```python
from build123d import *

# Parameters (mm, degrees)
F1_DEPTH = 7.5
F2_R     = 4
F3_T     = -0.95


with BuildPart() as f1:
    # F0 (on Top) → F1 (new body)
    with BuildSketch(Plane.XY):
        Polygon((-11.2561800848, -12.5999993347), (14, -12.5999993347), (14, 2.4000006653), (14, 8.4000006653), (14, 12.4000006653), (-14, 12.4000006653), (-14, 5.4000006653), (-14, -12.5999993347), align=None)
        with BuildLine():
            ThreePointArc((2.6457513111, -8.5999993347), (0, -9.5999993347), (-2.6457513111, -8.5999993347))
            Line((-2.6457513111, -8.5999993347), (-5.3542486889, -8.5999993347))
            ThreePointArc((-5.3542486889, -8.5999993347), (-8, -9.5999993347), (-10.6457513111, -8.5999993347))
            ThreePointArc((-10.6457513111, -8.5999993347), (-12, -5.5999993347), (-10.6457513111, -2.5999993347))
            ThreePointArc((-10.6457513111, -2.5999993347), (-8, -1.5999993347), (-5.3542486889, -2.5999993347))
            Line((-5.3542486889, -2.5999993347), (-2.6457513111, -2.5999993347))
            ThreePointArc((-2.6457513111, -2.5999993347), (0, -1.5999993347), (2.6457513111, -2.5999993347))
            Line((2.6457513111, -2.5999993347), (5.3542486889, -2.5999993347))
            ThreePointArc((5.3542486889, -2.5999993347), (8, -1.5999993347), (10.6457513111, -2.5999993347))
            ThreePointArc((10.6457513111, -2.5999993347), (12, -5.5999993347), (10.6457513111, -8.5999993347))
            ThreePointArc((10.6457513111, -8.5999993347), (8, -9.5999993347), (5.3542486889, -8.5999993347))
            Line((5.3542486889, -8.5999993347), (2.6457513111, -8.5999993347))
        make_face(mode=Mode.SUBTRACT)
        with BuildLine():
            Line((-2.6457513111, 2.4000006653), (-5.3542486889, 2.4000006653))
            ThreePointArc((-5.3542486889, 2.4000006653), (-12, 5.4000006653), (-5.3542486889, 8.4000006653))
            Line((-5.3542486889, 8.4000006653), (-2.6457513111, 8.4000006653))
            ThreePointArc((-2.6457513111, 8.4000006653), (0, 9.4000006653), (2.6457513111, 8.4000006653))
            Line((2.6457513111, 8.4000006653), (5.3542486889, 8.4000006653))
            ThreePointArc((5.3542486889, 8.4000006653), (8, 9.4000006653), (10.6457513111, 8.4000006653))
            ThreePointArc((10.6457513111, 8.4000006653), (12, 5.4000006653), (10.6457513111, 2.4000006653))
            ThreePointArc((10.6457513111, 2.4000006653), (8, 1.4000006653), (5.3542486889, 2.4000006653))
            Line((5.3542486889, 2.4000006653), (2.6457513111, 2.4000006653))
            ThreePointArc((2.6457513111, 2.4000006653), (0, 1.4000006653), (-2.6457513111, 2.4000006653))
        make_face(mode=Mode.SUBTRACT)
    extrude(amount=F1_DEPTH)

    # F2
    f2_edges = [f1.edges().sort_by_distance(p)[0] for p in [
        (-14, 12.400001, 3.75),
        (14, -12.599999, 3.75),
        (-14, -12.599999, 3.75),
        (14, 12.400001, 3.75),
    ]]
    fillet(f2_edges, radius=F2_R)

    # F3
    f3_openings = [f1.faces().sort_by_distance(p)[0] for p in [
        (0, -0.099999, 7.5),
    ]]
    offset(amount=F3_T, openings=f3_openings)


solid = f1.part
```
Work out the finished part from the listing and answer in its coordinate system (mm). A direction names the side the tool comes from. Coordinates: 2 decimals unless noted, no trailing zeros. Write each loop counter-clockwise with the first axis right and the second up, starting at its lowest first coordinate (ties: lowest second). Pieces come first, ordered by that corner, then holes.
Q1. A cutting plane is placed at B-B, the plane x = -8. Give the vertices of the cut face in (y, z).
Q2. A cutting plane is placed at A-A, the plane y = 5.4. Give the vertices of the cut face in (x, z), then the cut area to 3 significant figures.
Q3. Find the intervals of material crossed by line 1 (Y direction, x = 7.75, z = 5); line 2 (Y direction, x = -4.5, z = 5.75); line 3 (X direction, y = -0.25, z = 3.5), in increasing order.
Q4. A cutting plane is placed at C-C, the plane z = 0.5. Give the vertices of the cut face in (x, y), then the cut area to 3 significant figures.
Q5. Determine the mould class of faces 4 (the face through (-12.133, -10.78, 4.271)), 5 (the face through (0, -10, 7.5)), 6 (the face through (-12.797, 11.259, 3.802)), 7 (the face through (4, 8.4, 4)) for opening direction Y: released by +Y, released by -Y, zero draft, split by the parting line, or undercut.
Q6. This flat-tipped pin is pushed along its axis until it touches: pin 1 Ø1.5 at (y, z) = (9.5, 2.5) entering from -X. Where does it stop, or does it pass through?
Q7. A cutting plane is placed at D-D, the plane z = 3.75. State how many separate pieces and enclosed holes the cut face has, then the cut area to 3 significant figures.
Q8. Which of the six approach directions +Z, -Z, +X, -X, +Y, -Y give full straight-line access (tool end or side, diameter ignored) to faces 1 (the face through (0, 0, 0)), 2 (the face through (-0.04, -0.65, 4.18)), 3 (the face through (-4, 8.4, 4))?
Findings below:
1. outline: (-12.6, 0) - (-9.6, 0) - (-9.6, 7.5) - (-10.55, 7.5) - (-10.55, 0.95) - (-11.65, 0.95) - (-11.65, 7.5) - (-12.6, 7.5) - close; (-1.6, 0) - (1.4, 0) - (1.4, 7.5) - (0.45, 7.5) - (0.45, 0.95) - (-0.65, 0.95) - (-0.65, 7.5) - (-1.6, 7.5) - close; (9.4, 0) - (12.4, 0) - (12.4, 7.5) - (11.45, 7.5) - (11.45, 0.95) - (10.35, 0.95) - (10.35, 7.5) - (9.4, 7.5) - close
2. outline: (-14, 0) - (-12, 0) - (-12, 7.5) - (-12.95, 7.5) - (-12.95, 0.95) - (-13.05, 0.95) - (-13.05, 7.5) - (-14, 7.5) - close; (12, 0) - (14, 0) - (14, 7.5) - (13.05, 7.5) - (13.05, 0.95) - (12.95, 0.95) - (12.95, 7.5) - (12, 7.5) - close
2. area: 28.7 mm2
3. line 1: y = -12.6 to -11.65, -10.54 to -9.59, -1.61 to -0.66, 0.46 to 1.41, 9.39 to 10.34, 11.45 to 12.4
3. line 2: y = -12.6 to -11.65, -9.55 to -8.6, -2.6 to -1.65, 1.45 to 2.4, 8.4 to 9.35, 11.45 to 12.4
3. line 3: x = -14 to -13.05, 13.05 to 14
4. outline: (-14, -8.6) arc R4 ccw to (-10, -12.6) - (10, -12.6) arc R4 ccw to (14, -8.6) - (14, 8.4) arc R4 ccw to (10, 12.4) - (-10, 12.4) arc R4 ccw to (-14, 8.4) - close; hole (-5.35, -8.6) - (-2.65, -8.6) arc R4 ccw to (2.65, -8.6) - (5.35, -8.6) arc R4 ccw (long way) to (5.35, -2.6) - (2.65, -2.6) arc R4 ccw to (-2.65, -2.6) - (-5.35, -2.6) arc R4 ccw (long way) to start; hole (-5.35, 2.4) - (-2.65, 2.4) arc R4 ccw to (2.65, 2.4) - (5.35, 2.4) arc R4 ccw (long way) to (5.35, 8.4) - (2.65, 8.4) arc R4 ccw to (-2.65, 8.4) - (-5.35, 8.4) arc R4 ccw (long way) to start
4. area: 365 mm2
5. face 4: undercut
5. face 5: zero draft
5. face 6: released by +Y
5. face 7: undercut
6. pin 1: stops at x = -13.98
7. separate pieces: 3
7. enclosed holes: 3
7. area: 209 mm2
8. face 1: -Z, +X, -X, +Y, -Y
8. face 2: +Z
8. face 3: +Z, -Z
